Read the model definition and answer for the solid it produces. Units are mm, in the model's axes. A direction names the side the tool comes from. Coordinates: 2 decimals unless noted, no trailing zeros. Write each loop counter-clockwise with the first axis right and the second up, starting at its lowest first coordinate (ties: lowest second). Pieces come first, ordered by that corner, then holes. Notation, with made-up numbers: (54, 85) -> (110, 85) arc R15 cw to (110, 104) -> close; hole circle Ø5 at (88.5, 11). An arc over 180 degrees is marked (long way). Answer in a Markdown table with one row per item. Add a question column.
Item 1: Section A-A on z = -14 is taken. Write down the section's boundary in (x, y).
Item 2: Section C-C on x = 1.6 is taken. Count the separate pieces of the cut face and the enclosed holes in it, then the cut area to 3 significant figures.
Item 3: Section B-B on y = -45 is taken. Write down the section's boundary in (x, z).
Item 4: Straight lines are drawn through the part: line 1 (Y direction, x = 1.6, z = -208); line 2 (Y direction, x = 2.4, z = -166); line 3 (Z direction, x = 1.3, y = -47.5). For each, find the intervals that lie inside material, in ascending order. Write a range as from..to.
Item 5: Section D-D on z = -65 is taken. Write down the section's boundary in (x, y).
Item 6: Which of the six approach directions +Z, -Z, +X, -X, +Y, -Y give full straight-line access (tool end or side, diameter ignored) to faces 3 (the face through (1.479, -20.257, -35.6)), 4 (the face through (3, -13, -122))?
Item 7: For a pull along Y with two mould halves and no side action, classify faces 1 (the face through (1.479, 11.762, -9.418)), 2 (the face through (0, -13, -122)) as +Y half, -Y half, draft (parallel to the pull), parting line (faces both ways), or undercut.
```python
from build123d import *

# Parameters (mm, degrees)
SKETCH_1_W           = 290
SKETCH_1_H           = 120
EXTRUDE_1_DEPTH      = 3
CUT_EXTRUDE_5_DEPTH  = 10
CUT_EXTRUDE_6_DEPTH  = 3
SKETCH_4_W           = 45
SKETCH_4_H           = 35
CUT_EXTRUDE_10_DEPTH = 10
CUT_EXTRUDE_11_DEPTH = 3
CUT_EXTRUDE_12_DEPTH = 3
SKETCH_7_R           = 4.5
CUT_EXTRUDE_13_DEPTH = 3


with BuildPart() as part:
    # Sketch 1 → Extrude 1 (new body)
    with BuildSketch(Plane(origin=(0, 0, 0), x_dir=(0, 0, -1), z_dir=(1, 0, 0))):
        with Locations((124.096517683, -26.682755594)):
            Rectangle(SKETCH_1_W, SKETCH_1_H)
    extrude(amount=EXTRUDE_1_DEPTH)

    # Sketch 2 → Cut-Extrude 5 (cut)
    with BuildSketch(Plane.ZY):
        with BuildLine():
            Line((-79.096517683, -16.682755594), (-44.096517683, -16.682755594))
            ThreePointArc((-44.096517683, -16.682755594), (-42.632051589, -13.147221688), (-39.096517683, -11.682755594))
            Line((-39.096517683, -11.682755594), (-39.096517683, 23.317244406))
            ThreePointArc((-39.096517683, 23.317244406), (-67.38078893, 11.601515654), (-79.096517683, -16.682755594))
        make_face()
        with BuildLine():
            Line((-34.096517683, -16.682755594), (0.903482317, -16.682755594))
            ThreePointArc((0.903482317, -16.682755594), (-10.812246435, -44.967026841), (-39.096517683, -56.682755594))
            Line((-39.096517683, -56.682755594), (-39.096517683, -21.682755594))
            ThreePointArc((-39.096517683, -21.682755594), (-35.560983777, -20.2182895), (-34.096517683, -16.682755594))
        make_face()
    extrude(amount=-CUT_EXTRUDE_5_DEPTH, mode=Mode.SUBTRACT)

    # Sketch 3 → Cut-Extrude 6 (cut)
    with BuildSketch(Plane.ZY):
        with BuildLine():
            Line((-78.531190081, -21.204087707), (-43.506744141, -21.658309654))
            Line((-43.506744141, -21.658309654), (-43.960966088, -56.682755594))
            ThreePointArc((-43.960966088, -56.682755594), (-68.593950791, -46.103149466), (-78.531190081, -21.204087707))
        make_face()
        with BuildLine():
            Line((-34.265995521, 22.933541451), (-35.119719469, -12.186178019))
            Line((-35.119719469, -12.186178019), (0, -13.039901967))
            ThreePointArc((0, -13.039901967), (-9.682653686, 12.043539778), (-34.265995521, 22.933541451))
        make_face()
    extrude(amount=-CUT_EXTRUDE_6_DEPTH, mode=Mode.SUBTRACT)

    # Sketch 4 → Cut-Extrude 10 (cut)
    with BuildSketch(Plane.ZY):
        with Locations((-192.258808878, 5.817244406)):
            Rectangle(SKETCH_4_W, SKETCH_4_H)
        with Locations((-137.258808878, 5.817244406)):
            Rectangle(SKETCH_4_W, SKETCH_4_H)
        with Locations((-137.258808878, -39.182755594)):
            Rectangle(SKETCH_4_W, SKETCH_4_H)
        with Locations((-192.258808878, -39.182755594)):
            Rectangle(SKETCH_4_W, SKETCH_4_H)
    extrude(amount=-CUT_EXTRUDE_10_DEPTH, mode=Mode.SUBTRACT)

    # Sketch 5 → Cut-Extrude 11 (cut)
    with BuildSketch(Plane.ZY):
        with BuildLine():
            Line((-239.875713673, 22.237845944), (-239.875713673, -34.9202452))
            ThreePointArc((-239.875713673, -34.9202452), (-243.375713673, -38.4202452), (-246.875713673, -34.9202452))
            Line((-246.875713673, -34.9202452), (-246.875713673, 22.237845944))
            ThreePointArc((-246.875713673, 22.237845944), (-243.375713673, 25.737845944), (-239.875713673, 22.237845944))
        make_face()
        with BuildLine():
            Line((-225.875713673, 22.237845944), (-225.875713673, -34.9202452))
            ThreePointArc((-225.875713673, -34.9202452), (-229.375713673, -38.4202452), (-232.875713673, -34.9202452))
            Line((-232.875713673, -34.9202452), (-232.875713673, 22.237845944))
            ThreePointArc((-232.875713673, 22.237845944), (-229.375713673, 25.737845944), (-225.875713673, 22.237845944))
        make_face()
        with BuildLine():
            Line((-253.875713673, 22.237845944), (-253.875713673, -34.9202452))
            ThreePointArc((-253.875713673, -34.9202452), (-257.375713673, -38.4202452), (-260.875713673, -34.9202452))
            Line((-260.875713673, -34.9202452), (-260.875713673, 22.237845944))
            ThreePointArc((-260.875713673, 22.237845944), (-257.375713673, 25.737845944), (-253.875713673, 22.237845944))
        make_face()
    extrude(amount=-CUT_EXTRUDE_11_DEPTH, mode=Mode.SUBTRACT)

    # Sketch 6 → Cut-Extrude 12 (cut)
    with BuildSketch(Plane.ZY):
        with BuildLine():
            Line((-214.758808878, -65.609469687), (-114.758808878, -65.609469687))
            ThreePointArc((-114.758808878, -65.609469687), (-110.758808878, -69.609469687), (-114.758808878, -73.609469687))
            Line((-114.758808878, -73.609469687), (-214.758808878, -73.609469687))
            ThreePointArc((-214.758808878, -73.609469687), (-218.758808878, -69.609469687), (-214.758808878, -65.609469687))
        make_face()
        with BuildLine():
            Line((-98.541599086, 23.317244406), (-98.541599086, -56.682755594))
            ThreePointArc((-98.541599086, -56.682755594), (-102.541599086, -60.682755594), (-106.541599086, -56.682755594))
            Line((-106.541599086, -56.682755594), (-106.541599086, 23.317244406))
            ThreePointArc((-106.541599086, 23.317244406), (-102.541599086, 27.317244406), (-98.541599086, 23.317244406))
        make_face()
        with BuildLine():
            Line((0.903482317, -73.609469687), (-78.534135294, -73.609469687))
            ThreePointArc((-78.534135294, -73.609469687), (-82.534135294, -69.609469687), (-78.534135294, -65.609469687))
            Line((-78.534135294, -65.609469687), (0.903482317, -65.609469687))
            ThreePointArc((0.903482317, -65.609469687), (4.903482317, -69.609469687), (0.903482317, -73.609469687))
        make_face()
    extrude(amount=-CUT_EXTRUDE_12_DEPTH, mode=Mode.SUBTRACT)

    # Sketch 7 → Cut-Extrude 13 (cut)
    with BuildSketch(Plane.ZY):
        with BuildLine():
            ThreePointArc((-246.096517683, -72.501000298), (-250.596517683, -68.001000298), (-246.096517683, -63.501000298))
            Line((-246.096517683, -63.501000298), (-269.096517683, -63.501000298))
            Line((-269.096517683, -63.501000298), (-269.096517683, -72.501000298))
            Line((-269.096517683, -72.501000298), (-246.096517683, -72.501000298))
        make_face()
        with Locations((-246.096517683, -68.001000298)):
            Circle(SKETCH_7_R)
    extrude(amount=-CUT_EXTRUDE_13_DEPTH, mode=Mode.SUBTRACT)


solid = part.part
```
Results below:
| question | item | result |
|---|---|---|
| 1 | outline | (0, -86.68) -> (3, -86.68) -> (3, -73.61) -> (0, -73.61) -> close; (0, -65.61) -> (3, -65.61) -> (3, -47.83) -> (0, -47.83) -> close; (0, -16.68) -> (3, -16.68) -> (3, -12.7) -> (0, -12.7) -> close; (0, 15.89) -> (3, 15.89) -> (3, 33.32) -> (0, 33.32) -> close |
| 2 | separate pieces | 1 |
| 2 | enclosed holes | 14 |
| 2 | area | 20,300 mm2 |
| 3 | outline | (0, -269.1) -> (3, -269.1) -> (3, -214.76) -> (0, -214.76) -> close; (0, -169.76) -> (3, -169.76) -> (3, -159.76) -> (0, -159.76) -> close; (0, -114.76) -> (3, -114.76) -> (3, -106.54) -> (0, -106.54) -> close; (0, -98.54) -> (3, -98.54) -> (3, -69.62) -> (0, -69.62) -> close; (0, -43.81) -> (3, -43.81) -> (3, -39.1) -> (0, -39.1) -> close; (0, -10.85) -> (3, -10.85) -> (3, 20.9) -> (0, 20.9) -> close |
| 4 | line 1 | y = -86.68..-73.61, -65.61..-56.68, -21.68..-11.68, 23.32..33.32 |
| 4 | line 2 | y = -86.68..-73.61, -65.61..33.32 |
| 4 | line 3 | z = -269.1..-214.76, -169.76..-159.76, -114.76..-106.54, -98.54..-67.15, -43.84..-39.1, -13.6..20.9 |
| 5 | outline | (0, -86.68) -> (3, -86.68) -> (3, -73.61) -> (0, -73.61) -> close; (0, -65.61) -> (3, -65.61) -> (3, -49.32) -> (0, -49.32) -> close; (0, -21.38) -> (3, -21.38) -> (3, -16.68) -> (0, -16.68) -> close; (0, 13.8) -> (3, 13.8) -> (3, 33.32) -> (0, 33.32) -> close |
| 6 | face 3 | +X, -X |
| 6 | face 4 | +Z, -Z, +X, +Y, -Y |
| 7 | face 1 | undercut |
| 7 | face 2 | draft |
